from build123d import *

# Parameters (mm, degrees)
SKETCH1_W           = 83.82
SKETCH1_H           = 12.7
SKETCH1_R           = 2.286
BOSS_EXTRUDE1_DEPTH = 25.4
SKETCH2_R           = 2.286
CUT_EXTRUDE1_DEPTH  = 12.7
FILLET1_R           = 2.54
SKETCH3_W           = 71.12
SKETCH3_H           = 19.05
CUT_EXTRUDE2_DEPTH  = 89.499957062
CHAMFER1_SIZE       = 19.55628504
CHAMFER1_SIZE_2     = 12.7
FILLET2_R           = 2.54


with BuildPart() as part:
    # Sketch1 → Boss-Extrude1 (new body)
    with BuildSketch(Plane(origin=(0, 0, 0), x_dir=(1, 0, 0), z_dir=(0, 1, 0))):
        with Locations((41.91, 6.35)):
            Rectangle(SKETCH1_W, SKETCH1_H)
        with Locations(Location((6.35, 6.35, 0), (0, 0, 90))):
            Circle(SKETCH1_R, mode=Mode.SUBTRACT)
        with Locations(Location((47.659178157, 6.35, 0), (0, 0, 90))):
            Circle(SKETCH1_R, mode=Mode.SUBTRACT)
    extrude(amount=BOSS_EXTRUDE1_DEPTH)

    # Sketch2 → Cut-Extrude1 (cut)
    with BuildSketch(Plane.XY):
        with Locations((77.47, 19.05)):
            Circle(SKETCH2_R)
    extrude(amount=-CUT_EXTRUDE1_DEPTH, mode=Mode.SUBTRACT)

    # Fillet1
    fillet1_edges = [part.edges().sort_by_distance(p)[0] for p in [
        (0, 12.7, -12.7),
        (83.82, 12.7, -12.7),
        (83.82, 12.7, 0),
        (0, 12.7, 0),
    ]]
    fillet(fillet1_edges, radius=FILLET1_R)

    # Sketch3 → Cut-Extrude2 (cut, through all)
    with BuildSketch(Plane.XY):
        with Locations((35.56, 15.875)):
            Rectangle(SKETCH3_W, SKETCH3_H)
    extrude(amount=-CUT_EXTRUDE2_DEPTH, mode=Mode.SUBTRACT)

    # Chamfer1
    # the kernel refuses this chamfer: 19.55628504, 12.7 mm, written as the material it adds along each edge
    with BuildSketch(Plane(origin=(71.12, 6.35, 0), x_dir=(0.021073765466273545, 0.9997779235455604, 0), z_dir=(0, 0, -1))) as chamfer1_piece_1_section:
        Polygon((CHAMFER1_SIZE * 0.999777923568, -CHAMFER1_SIZE * 0.0210737654668), (-CHAMFER1_SIZE_2 * 0.0210737654663, -CHAMFER1_SIZE_2 * 0.999777923546), (0, 0), align=None)
    chamfer1_piece_1 = extrude(amount=12.7, mode=Mode.PRIVATE)
    chamfer1_piece_1 = split(chamfer1_piece_1, bisect_by=Plane(origin=(66.98884067, 25.4, -6.35), z_dir=(0, -1, 0)), keep=Keep.TOP, mode=Mode.PRIVATE)
    add(chamfer1_piece_1)

    # Fillet2
    fillet2_edges = [part.edges().sort_by_distance(p)[0] for p in [
        (76.035607325, 25.4, -12.7),
        (83.82, 25.4, -6.35),
        (83.076051224, 25.4, -0.743948776),
        (83.076051224, 25.4, -11.956051224),
        (0.743948776, 6.35, -0.743948776),
        (76.035607325, 25.4, 0),
        (0, 6.35, -6.35),
        (0.743948776, 6.35, -11.956051224),
        (30.48, 6.35, -12.7),
        (30.48, 6.35, 0),
        (58.42, 6.35, -6.35),
        (70.79121465, 25.4, -6.35),
        (64.605607325, 15.875, 0),
        (64.605607325, 15.875, -12.7),
    ]]
    fillet(fillet2_edges, radius=FILLET2_R)


solid = part.part
The model under review builds one solid part; all positions refer to its coordinate system, in mm. A direction names the side the tool comes from. Round coordinates to 2 decimals unless told otherwise and drop trailing zeros. Write each loop counter-clockwise with the first axis right and the second up, starting at its lowest first coordinate (ties: lowest second). Pieces come first, ordered by that corner, then holes. Notation, with made-up numbers: M -38,9 L -2,9 A28 cw -2,40 Z; hole C 69,11.25 d6. An arc over 180 degrees is marked long. Answer as CSV lines item,"result". Start each with the question number.
Q1. Tool access review of faces 5 (the face through (29.409, 5.586, -11.976)), 6 (the face through (41, 0, -6)): name each direction out of +Z, -Z, +X, -X, +Y, -Y from which nothing blocks a thin tool from reaching the whole face with its end or side.
Q2. Consider section B-B, the plane x = 6.35. Give the boundary of the cut face in (y, z).
Q3. The part is to be moulded in two halves that separate along X. For faces 1 (the face through (45.73, 3.13, -7.58)), 2 (the face through (83.056, 24.676, -6.297)), 3 (the face through (0.724, 1.932, -11.936)), 4 (the face through (77, 25.4, -6)), say which applies: +X half, -X half, draft (parallel to the pull), parting line (faces both ways), or undercut.
Q4. Wall thickness on line 1 along X through (y, z) = (4, -6.35); line 2 along Y through (x, z) = (77.47, -5.25); line 3 along X through (y, z) = (4.75, -6.35): over which ranges is each line inside the solid? List them lowest first.
Q5. Clearance check with flat-ended pins moving along their axes: P1, Ø5, axis at x = 9, z = -6.5, coming from the +Y side; P2, Ø5, axis at y = 11.5, z = -6, coming from the -X side; P3, Ø1, axis at y = 21, z = -10.5, coming from the +X side. State where each tip first meets the part, or that it passes through.
Q6. Consider section A-A, the plane z = -6.35. Give the boundary of the cut face in (x, y), then the cut area to 3 significant figures.
Q7. Consider section C-C, the plane z = -1.25. Give the boundary of the cut face in (x, y).
Q8. Consider section D-D, the plane y = 5.25. State how many separate pieces and enclosed holes the cut face has, then the cut area to 3 significant figures.
Result set:
1,face 5,"-Z, -X, +Y"
1,face 6,"+Z, -Z, +X, -X, -Y"
2,outline,"M 0,-12.7 L 3.81,-12.7 A2.54 ccw 6.35,-10.16 L 6.35,-8.64 L 0,-8.64 Z; M 0,-4.06 L 6.35,-4.06 L 6.35,-2.54 A2.54 ccw 3.81,0 L 0,0 Z"
3,face 1,"undercut"
3,face 2,"+X half"
3,face 3,"-X half"
3,face 4,"draft"
4,line 1,"x = 0.01 to 4.06, 8.64 to 45.37, 49.95 to 83.82"
4,line 2,"y = 0 to 16.76, 21.34 to 25.4"
4,line 3,"x = 0.18 to 4.06, 8.64 to 45.37, 49.95 to 83.82"
5,P1,"stops at y = 6.35"
5,P2,"stops at x = 60.14"
5,P3,"stops at x = 83.82"
6,outline,"M 0,0 L 4.06,0 L 4.06,6.35 L 2.54,6.35 A2.54 ccw 0,3.81 Z; M 8.64,0 L 45.37,0 L 45.37,6.35 L 8.64,6.35 Z; M 49.95,0 L 83.82,0 L 83.82,22.86 A2.54 ccw 81.28,25.4 L 72.17,25.4 A2.54 ccw 70.04,24.24 L 59.17,7.51 A2.54 cw 57.04,6.35 L 49.95,6.35 Z; hole C 77.47,19.05 d4.57"
6,area,"821 mm²"
7,outline,"M 0.35,0 L 83.47,0 L 83.47,22.86 A2.19 ccw 81.28,25.05 L 72.17,25.05 A2.19 ccw 70.34,24.05 L 59.47,7.31 A2.89 cw 57.04,6 L 2.54,6 A2.19 ccw 0.35,3.81 Z; hole C 77.47,19.05 d4.57"
8,separate pieces,"1"
8,enclosed holes,"2"
8,area,"969 mm²"
